```python
from build123d import *

# Parameters (mm, degrees)
PAD_DEPTH    = 160
SKETCH001_W  = 23.4827
SKETCH001_H  = 25.6175
POCKET_DEPTH = 29.1745


with BuildPart() as part:
    # Sketch → Pad (new body)
    with BuildSketch(Plane.XY):
        with BuildLine():
            Line((0.060026, 0.138063), (29.233526, 0.138063))
            Line((29.233526, 0.138063), (29.233526, -49.804137))
            ThreePointArc((0.060026, -53.095937), (15.982721, -63.289822), (29.233526, -49.804137))
            Line((0.060026, -53.095937), (0.060026, 0.138063))
        make_face()
    extrude(amount=PAD_DEPTH)

    # Sketch001 → Pocket (cut, through all)
    with BuildSketch(Plane.YZ.offset(29.233526)):
        with Locations((-25.419298, 80.703762)):
            Rectangle(SKETCH001_W, SKETCH001_H)
    extrude(amount=-POCKET_DEPTH, mode=Mode.SUBTRACT)


solid = part.part
```
Build history of the part. All positions in model axes, mm. A direction names the side the tool comes from. Round coordinates to 2 decimals unless told otherwise and drop trailing zeros. Loops run counter-clockwise (first coordinate to the right, second up) from the corner with the lowest first, then second, coordinate; pieces in that order, holes last.
Item 1: Saw through at C-C (x = 20.75). List the corners of the cut face in (y, z), then the cut area to 3 significant figures.
Item 2: Which spindle directions (+Z, -Z, +X, -X, +Y, -Y) get a long thin tool onto all of the face, cutting with end or side? Do faces 1 (the face through (14, 0.138, 79)), 2 (the face through (15, -26, 93.513)). Say none if no direction does.
Item 3: Saw through at B-B (y = -21.5). List the corners of the cut face in (x, z).
Item 4: Pin check, flat tips, straight feed: P1, Ø10, axis at x = 8.5, z = 56.5, coming from the -Y side; P2, Ø3, axis at x = 22, z = 130, coming from the -Y side; P3, Ø8, axis at x = 24, y = -42, coming from the -Z side. Stop position of each tip, or through.
Item 5: Saw through at A-A (z = 70). List the corners of the cut face in (x, y).
Item 6: Drill centre lines: line 1 along Z through (x, y) = (15.5, -34); line 2 along Y through (x, z) = (8.25, 86.5); line 3 along Y through (x, z) = (10.75, 77). Where is each one in solid material? Low to high.
Item 7: Saw through at D-D (x = 3). List the corners of the cut face in (y, z), then the cut area to 3 significant figures.
Item 8: Two-plate mould, pull along Z, no slides. Class faces 3 (the face through (15.7, -63.32, 78.88)), 4 (the face through (15, -31, 160)), 5 (the face through (15, -13.678, 81)): released by +Z, released by -Z, zero draft, split by the parting line, or undercut.
Worked answers:
1. outline: (-61.93, 0) - (0.14, 0) - (0.14, 160) - (-61.93, 160) - close; hole (-37.16, 67.9) - (-13.68, 67.9) - (-13.68, 93.51) - (-37.16, 93.51) - close
1. area: 9,330 mm2
2. face 1: +Z, -Z, +X, -X, +Y
2. face 2: +X, -X
3. outline: (0.06, 0) - (29.23, 0) - (29.23, 67.9) - (0.06, 67.9) - close; (0.06, 93.51) - (29.23, 93.51) - (29.23, 160) - (0.06, 160) - close
4. P1: stops at y = -63.36
4. P2: stops at y = -62.04
4. P3: stops at z = 0
5. outline: (0.06, -53.1) arc R15 ccw to (29.23, -49.8) - (29.23, -37.16) - (0.06, -37.16) - close; (0.06, -13.68) - (29.23, -13.68) - (29.23, 0.14) - (0.06, 0.14) - close
6. line 1: z = 0 to 67.9, 93.51 to 160
6. line 2: y = -62.11 to -37.16, -13.68 to 0.14
6. line 3: y = -62.96 to -37.16, -13.68 to 0.14
7. outline: (-58.25, 0) - (0.14, 0) - (0.14, 160) - (-58.25, 160) - close; hole (-37.16, 67.9) - (-13.68, 67.9) - (-13.68, 93.51) - (-37.16, 93.51) - close
7. area: 8,740 mm2
8. face 3: zero draft
8. face 4: released by +Z
8. face 5: undercut
